Build history of the part. All positions in model axes, mm. Round coordinates to 2 decimals unless told otherwise and drop trailing zeros. Loops run counter-clockwise (first coordinate to the right, second up) from the corner with the lowest first, then second, coordinate; pieces in that order, holes last.
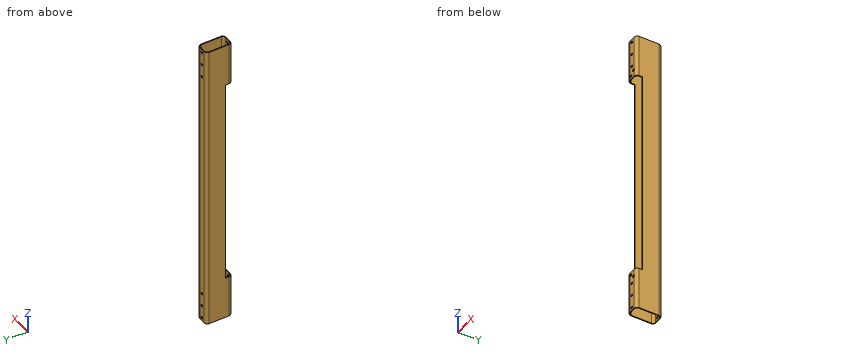
from build123d import *

# Parameters (mm, degrees)
EXTRUDE_THIN1_DEPTH               = 571.5
F_3_16_0_1875_DIAMETER_HOLE1_D    = 4.7625
SKETCH5_W                         = 406.4
SKETCH5_H                         = 12.7
CUT_EXTRUDE1_DEPTH                = 573.627776134
F_3_16_0_195_DIAMETER_HOLE1_D     = 4.953
F_3_16_0_195_DIAMETER_HOLE1_DEPTH = 25.4
F_3_16_0_195_DIAMETER_HOLE1_TIP   = 1.488031323


with BuildPart() as part:
    # Sketch1 → Extrude-Thin1 (new body)
    with BuildSketch(Plane.XY):
        with BuildLine():
            Line((-12.7, 19.05), (-12.7, -19.05))
            ThreePointArc((-12.7, -19.05), (-10.840128061, -23.540128061), (-6.35, -25.4))
            Line((-6.35, -25.4), (6.35, -25.4))
            ThreePointArc((6.35, -25.4), (10.840128061, -23.540128061), (12.7, -19.05))
            Line((12.7, -19.05), (12.7, 19.05))
            ThreePointArc((12.7, 19.05), (10.840128061, 23.540128061), (6.35, 25.4))
            Line((6.35, 25.4), (-6.35, 25.4))
            ThreePointArc((-6.35, 25.4), (-10.840128061, 23.540128061), (-12.7, 19.05))
        make_face()
        with BuildLine():
            Line((-11.1125, 19.05), (-11.1125, -19.05))
            ThreePointArc((-11.1125, -19.05), (-9.717596045, -22.417596045), (-6.35, -23.8125))
            Line((-6.35, -23.8125), (6.35, -23.8125))
            ThreePointArc((6.35, -23.8125), (9.717596045, -22.417596045), (11.1125, -19.05))
            Line((11.1125, -19.05), (11.1125, 19.05))
            ThreePointArc((11.1125, 19.05), (9.717596045, 22.417596045), (6.35, 23.8125))
            Line((6.35, 23.8125), (-6.35, 23.8125))
            ThreePointArc((-6.35, 23.8125), (-9.717596045, 22.417596045), (-11.1125, 19.05))
        make_face(mode=Mode.SUBTRACT)
    extrude(amount=EXTRUDE_THIN1_DEPTH)

    # 3/16 (0.1875) Diameter Hole1 (through all)
    with Locations(Plane(origin=(0, 25.4, 565.15), x_dir=(0, 0, 1), z_dir=(0, 1, 0))):
        with Locations((0, 0), (-558.8, 0), (-533.4, 0), (-508, 0), (-25.4, 0), (-50.8, 0)):
            Hole(F_3_16_0_1875_DIAMETER_HOLE1_D / 2)

    # Sketch5 → Cut-Extrude1 (cut, through all)
    with BuildSketch(Plane(origin=(12.7, 0, 0), x_dir=(0, 0, -1), z_dir=(1, 0, 0))):
        with Locations((-285.75, -19.05)):
            Rectangle(SKETCH5_W, SKETCH5_H)
    extrude(amount=-CUT_EXTRUDE1_DEPTH, mode=Mode.SUBTRACT)

    # 3/16 (0.195) Diameter Hole1
    with Locations(Plane(origin=(0, -25.4, 0), x_dir=(-1, 0, 0), z_dir=(0, -1, 0))):
        with Locations((2.54, -495.3), (-5.08, -502.92), (-5.08, -68.58), (2.54, -76.2)):
            Hole(F_3_16_0_195_DIAMETER_HOLE1_D / 2, depth=F_3_16_0_195_DIAMETER_HOLE1_DEPTH)
            with Locations((0, 0, -(F_3_16_0_195_DIAMETER_HOLE1_DEPTH + F_3_16_0_195_DIAMETER_HOLE1_TIP / 2))):  # 118° drill point
                Cone(0, F_3_16_0_195_DIAMETER_HOLE1_D / 2, F_3_16_0_195_DIAMETER_HOLE1_TIP, mode=Mode.SUBTRACT)


solid = part.part
(1) Probe line 1 (Z direction, x = 5.08, y = -24.55); line 2 (Z direction, x = -2.54, y = -24.6); line 3 (X direction, y = 4, z = 489). List the from-to ranges inside material, lowest first.
Responses:
line 1: z = 0 to 66.1, 71.06 to 82.55, 488.95 to 500.44, 505.4 to 571.5
line 2: z = 0 to 73.72, 78.68 to 82.55, 488.95 to 492.82, 497.78 to 571.5
line 3: x = -12.7 to -11.11, 11.11 to 12.7
(2) Pin check, flat tips, straight feed: P1, Ø4.5, axis at x = 0, z = 565.15, coming from the -Y side; P2, Ø6, axis at x = 0, z = 6.35, coming from the -Y side; P3, Ø2, axis at x = -9, z = 90.5, coming from the +Y side; P4, Ø6, axis at x = 2.5, z = 127, coming from the -Y side. Stop position of each tip, or through.
Responses:
P1: passes through
P2: stops at y = -25.4
P3: stops at y = 25.18
P4: stops at y = 23.81
(3) Slice it at A-A on y = 0.5. List the corners of the cut face in (x, z), plus the area to 3 significant figures.
Responses:
outline: (-12.7, 0) - (-11.11, 0) - (-11.11, 571.5) - (-12.7, 571.5) - close; (11.11, 0) - (12.7, 0) - (12.7, 571.5) - (11.11, 571.5) - close
area: 1,810 mm2
